Design review of the part shown in the three views and the two pictorial views. Dimensions are in mm from the part's minimum x, y and z. A direction names the side the tool comes from. Round coordinates to 2 decimals unless told otherwise and drop trailing zeros. Order: outer loops, then holes, each group sorted by start corner. A loop starts at its lowest first (then second) coordinate and runs counter-clockwise, first axis right, second up. Notation, with made-up numbers: M -36,83.5 L -18,83.5 A21 cw -18,96.5 Z; hole C -2,-4.75 d4. An arc over 180 degrees is marked long. Use a Markdown table: item, result. Add a question column.
(1) Take a section at C-C (z = 6). Write out the cut boundary in (x, y).
(2) For pin 1 (0.6 mm diameter, centred on x = 2, z = 0, fed in from -Y); pin 2 (1.5 mm diameter, centred on x = 3, z = 6, fed in from -Y); pin 3 (0.6 mm diameter, centred on y = 1, z = 0, fed in from +X) (1 decimal), all flat-tipped, find the tip position at first contact; note any pin that passes through.
(3) Machinability: for the marked faces 3 and 4, which of the approach directions +Z, -Z, +X, -X, +Y, -Y give a long, thin tool a straight path to every point of the face, cutting with its end or side? Answer none if there is none.
(4) To check wall thickness, follow probe 1 along Z at (x, y) = (2.9, 3.25); probe 2 along Z at (x, y) = (2.1, 1.35); probe 3 along Y at (x, z) = (1.35, 6.75). State the ranges of each line that lie inside material, in increasing order. Write a range as from..to.
(5) Take a section at A-A (x = 2). Write out the cut boundary in (y, z).
(6) The part is to be moulded in two halves that separate along X. For the marked faces 1 and 2, say which applies: released by +X, released by -X, zero draft, split by the parting line, or undercut.
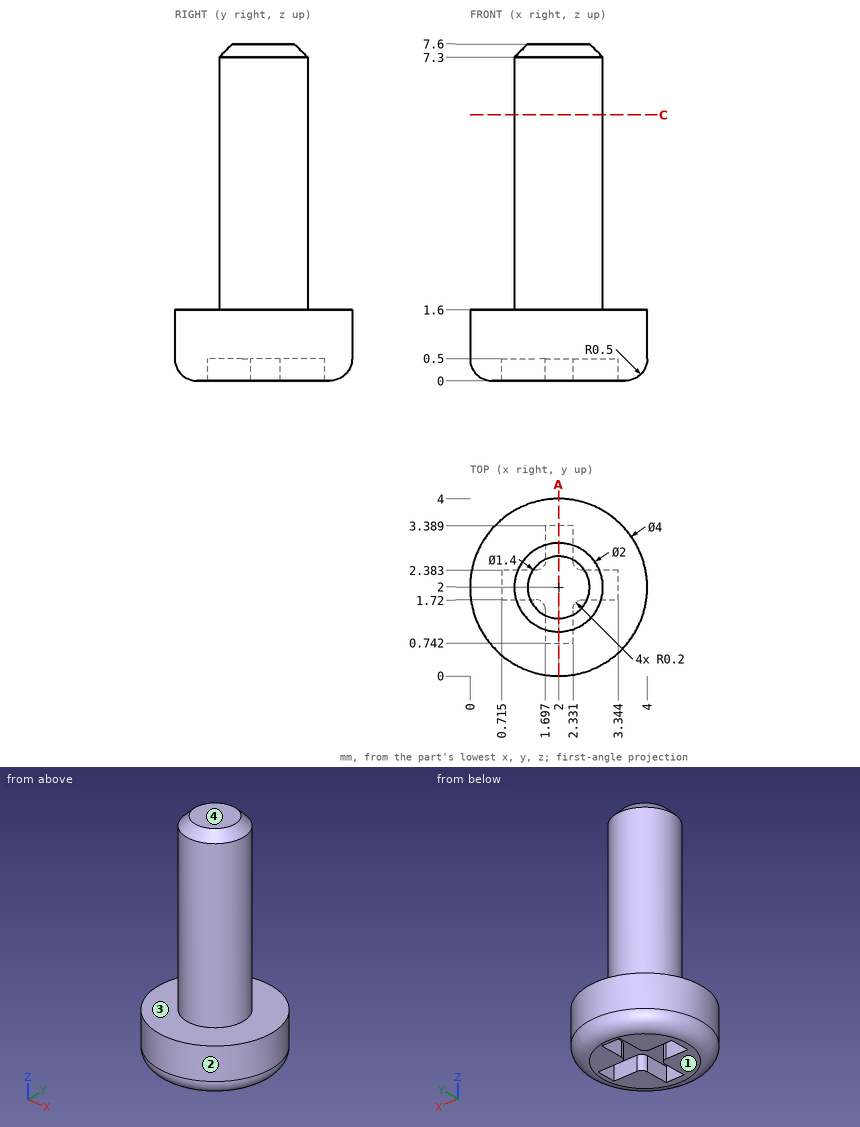
Verdict:
| question | item | result |
|---|---|---|
| 1 | outline | C 2,2 d2 |
| 2 | pin 1 | stops at y = 0.04 |
| 2 | pin 2 | stops at y = 1.03 |
| 2 | pin 3 | stops at x = 3.7 |
| 3 | face 3 | +Z |
| 3 | face 4 | +Z, +X, -X, +Y, -Y |
| 4 | probe 1 | z = 0..1.6 |
| 4 | probe 2 | z = 0.5..7.6 |
| 4 | probe 3 | y = 1.24..2.76 |
| 5 | outline | M 0,0.5 A0.5 ccw 0.5,0 L 0.74,0 L 0.74,0.5 L 3.39,0.5 L 3.39,0 L 3.5,0 A0.5 ccw 4,0.5 L 4,1.6 L 3,1.6 L 3,7.3 L 2.7,7.6 L 1.3,7.6 L 1,7.3 L 1,1.6 L 0,1.6 Z |
| 6 | face 1 | zero draft |
| 6 | face 2 | split by the parting line |
